Verification items for the finished model (mm, model axes). Face numbers are marked on the shaded views. A direction names the side the tool comes from. Round coordinates to 2 decimals unless told otherwise and drop trailing zeros. Write each loop counter-clockwise with the first axis right and the second up, starting at its lowest first coordinate (ties: lowest second). Pieces come first, ordered by that corner, then holes. Notation, with made-up numbers: (48.5, 85.25) - (106.5, 85.25) arc R27 ccw to (106.5, 118.25) - close; hole circle Ø4 at (24, 41). An arc over 180 degrees is marked (long way). Answer as a JSON object with one key per item and string values. Group by question number.
1) Section check A-A (y = 35). Enter the section's corners in (x, z).
2) Thickness scan on line 1 (X direction, y = 65, z = 3.25); line 2 (Y direction, x = 58, z = 3); line 3 (Y direction, x = -76, z = 10). Record the ranges inside material, lowest first.
3) Mould release check, pull along X, two halves, no side actions. Record for the marked faces 4, 5 and 6: +X half, -X half, draft (parallel to the pull), parting line (faces both ways), or undercut.
4) Section check B-B (x = 58). State how many separate pieces and enclosed holes the cut face has, then the cut area to 3 significant figures.
5) Go/stop test with flat-tipped pins: pin 1 Ø11.5 at (x, y) = (16, 79) entering from +Z; pin 2 Ø6.5 at (x, y) = (16, -43) entering from -Z; pin 3 Ø9 at (y, z) = (-80, 10) entering from +X. Record where each tip stops, or that it passes through.
6) Set-up check for the marked faces 1, 2 and 3: record each of +Z, -Z, +X, -X, +Y, -Y from which the full face is reachable in a straight line by a thin tool's end or side.
```python
from build123d import *

# Parameters (mm, degrees)
SKETCH_1_W                   = 186
SKETCH_1_H                   = 200
EXTRUDE_1_DEPTH              = 20
HOLE_WIZARD_M12_1_AT_2_COUNT = 2
HOLE_WIZARD_M12_1_AT_2_PITCH = 80
HOLE_WIZARD_M12_1_AT_3_COUNT = 2
HOLE_WIZARD_M12_1_AT_3_PITCH = 160
SKETCH_4_W                   = 44
SKETCH_4_H                   = 200
CUT_EXTRUDE_1_DEPTH          = 2
HOLE_WIZARD_2_D              = 5.5
HOLE_WIZARD_2_CBORE_D        = 10
HOLE_WIZARD_2_CBORE_DEPTH    = 6.5
HOLE_WIZARD_2_2_D            = 6.6
HOLE_WIZARD_2_2_CBORE_D      = 11
HOLE_WIZARD_2_2_CBORE_DEPTH  = 6.8
HOLE_WIZARD_M4_1_D           = 3.3
HOLE_WIZARD_M4_1_DEPTH       = 10.1
HOLE_WIZARD_M4_1_TIP         = 0.991420021
CUT_EXTRUDE_2_DEPTH          = 139.018114753
HOLE_WIZARD_M4_2_D           = 3.3
HOLE_WIZARD_M4_2_DEPTH       = 10.1
HOLE_WIZARD_M4_2_TIP         = 0.991420021
HOLE_WIZARD_M3_1_D           = 2.5
HOLE_WIZARD_M3_1_DEPTH       = 7.5
HOLE_WIZARD_M3_1_TIP         = 0.751075774
HOLE_WIZARD_1_D              = 25
HOLE_WIZARD_M6_1_D           = 5


with BuildPart() as part:
    # 草图1 → 凸台-拉伸1 (new body)
    with BuildSketch(Plane.XY):
        Rectangle(SKETCH_1_W, SKETCH_1_H)
    extrude(amount=EXTRUDE_1_DEPTH)

    # 草图2 → M12 螺纹孔1 (revolve, cut)
    with BuildSketch(Plane(origin=(-93, 80, 10), x_dir=(0, 0, 1), z_dir=(0, 1, 0))):
        Polygon((0, 0), (0, 30.064389157), (5.1, 27), (5.1, 0), align=None)
    hole_wizard_m12_1 = revolve(axis=Axis((-99.35, 80, 10), (1, 0, 0)), mode=Mode.SUBTRACT)

    # M12 螺纹孔1 at 2: M12 螺纹孔1 ×2
    with Locations(*[(0, -i * HOLE_WIZARD_M12_1_AT_2_PITCH, 0) for i in range(1, HOLE_WIZARD_M12_1_AT_2_COUNT)]):
        add(hole_wizard_m12_1, mode=Mode.SUBTRACT)

    # M12 螺纹孔1 at 3: M12 螺纹孔1 ×2
    with Locations(*[(0, -i * HOLE_WIZARD_M12_1_AT_3_PITCH, 0) for i in range(1, HOLE_WIZARD_M12_1_AT_3_COUNT)]):
        add(hole_wizard_m12_1, mode=Mode.SUBTRACT)

    # 镜向1: M12 螺纹孔1 across plane
    add(hole_wizard_m12_1.mirror(Plane(origin=(0, 0, 0), x_dir=(0, 0, 1), z_dir=(1, 0, 0))), mode=Mode.SUBTRACT)

    # 镜向1 copy 1 sketch → 镜向1 copy 1 (revolve, cut)
    with BuildSketch(Plane(origin=(93, 0, 10), x_dir=(0, 0, 1), z_dir=(0, 1, 0))):
        Polygon((0, 0), (0, -30.064389157), (5.1, -27), (5.1, 0), align=None)
    revolve(axis=Axis((99.35, 0, 10), (1, 0, 0)), mode=Mode.SUBTRACT)

    # 镜向1 copy 2 sketch → 镜向1 copy 2 (revolve, cut)
    with BuildSketch(Plane(origin=(93, -80, 10), x_dir=(0, 0, 1), z_dir=(0, 1, 0))):
        Polygon((0, 0), (0, -30.064389157), (5.1, -27), (5.1, 0), align=None)
    revolve(axis=Axis((99.35, -80, 10), (1, 0, 0)), mode=Mode.SUBTRACT)

    # 草图4 → 切除-拉伸1 (cut)
    with BuildSketch(Plane.XY.offset(20)):
        Rectangle(SKETCH_4_W, SKETCH_4_H)
    extrude(amount=-CUT_EXTRUDE_1_DEPTH, mode=Mode.SUBTRACT)

    # Hole Wizard 2 (through all)
    with Locations(Plane(origin=(0, 0, 0), x_dir=(-1, 0, 0), z_dir=(0, 0, -1))):
        with Locations((16, 79), (16, 43), (-16, 43), (-16, 79), (-16, -79), (-16, -43), (16, -43), (16, -79)):
            CounterBoreHole(HOLE_WIZARD_2_D / 2, HOLE_WIZARD_2_CBORE_D / 2, HOLE_WIZARD_2_CBORE_DEPTH)

    # Hole Wizard 2 2 (through all)
    with Locations(Plane(origin=(0, 0, 0), x_dir=(-1, 0, 0), z_dir=(0, 0, -1))):
        with Locations((-58, 94), (-58, 55), (-58, 16), (-83, 55)):
            CounterBoreHole(HOLE_WIZARD_2_2_D / 2, HOLE_WIZARD_2_2_CBORE_D / 2, HOLE_WIZARD_2_2_CBORE_DEPTH)

    # M4 螺纹孔1
    with Locations(Plane(origin=(0, 100, 0), x_dir=(1, 0, 0), z_dir=(0, 1, 0))):
        with Locations((-80, -10), (80, -10)):
            Hole(HOLE_WIZARD_M4_1_D / 2, depth=HOLE_WIZARD_M4_1_DEPTH)
            with Locations((0, 0, -(HOLE_WIZARD_M4_1_DEPTH + HOLE_WIZARD_M4_1_TIP / 2))):  # 118° drill point
                Cone(0, HOLE_WIZARD_M4_1_D / 2, HOLE_WIZARD_M4_1_TIP, mode=Mode.SUBTRACT)

    # 草图11 → 切除-拉伸2 (cut, through all)
    with BuildSketch(Plane(origin=(0, 0, 0), x_dir=(-1, 0, 0), z_dir=(0, 0, -1))):
        with BuildLine():
            Line((-17, -24), (17, -24))
            ThreePointArc((17, -24), (20.535533906, -22.535533906), (22, -19))
            Line((22, -19), (22, 19))
            ThreePointArc((22, 19), (20.535533906, 22.535533906), (17, 24))
            Line((17, 24), (-17, 24))
            ThreePointArc((-17, 24), (-20.535533906, 22.535533906), (-22, 19))
            Line((-22, 19), (-22, -19))
            ThreePointArc((-22, -19), (-20.535533906, -22.535533906), (-17, -24))
        make_face()
    extrude(amount=-CUT_EXTRUDE_2_DEPTH, mode=Mode.SUBTRACT)

    # M4 螺纹孔2
    with Locations(Plane(origin=(0, 0, 0), x_dir=(-1, 0, 0), z_dir=(0, 0, -1))):
        with Locations((-12.5, 65), (12.5, 65)):
            Hole(HOLE_WIZARD_M4_2_D / 2, depth=HOLE_WIZARD_M4_2_DEPTH)
            with Locations((0, 0, -(HOLE_WIZARD_M4_2_DEPTH + HOLE_WIZARD_M4_2_TIP / 2))):  # 118° drill point
                Cone(0, HOLE_WIZARD_M4_2_D / 2, HOLE_WIZARD_M4_2_TIP, mode=Mode.SUBTRACT)

    # M3 螺纹孔1
    with Locations(Plane.XY.offset(20)):
        with Locations((-32, 70), (-32, -70), (-40, -70), (-40, 70)):
            Hole(HOLE_WIZARD_M3_1_D / 2, depth=HOLE_WIZARD_M3_1_DEPTH)
            with Locations((0, 0, -(HOLE_WIZARD_M3_1_DEPTH + HOLE_WIZARD_M3_1_TIP / 2))):  # 118° drill point
                Cone(0, HOLE_WIZARD_M3_1_D / 2, HOLE_WIZARD_M3_1_TIP, mode=Mode.SUBTRACT)

    # 孔1 (through all)
    with Locations(Plane.XY.offset(20)):
        with Locations((77, 35)):
            Hole(HOLE_WIZARD_1_D / 2)

    # M6 螺纹孔1 (through all)
    with Locations(Plane(origin=(0, 0, 0), x_dir=(-1, 0, 0), z_dir=(0, 0, -1))):
        with Locations((-58, 85)):
            Hole(HOLE_WIZARD_M6_1_D / 2)


solid = part.part
```
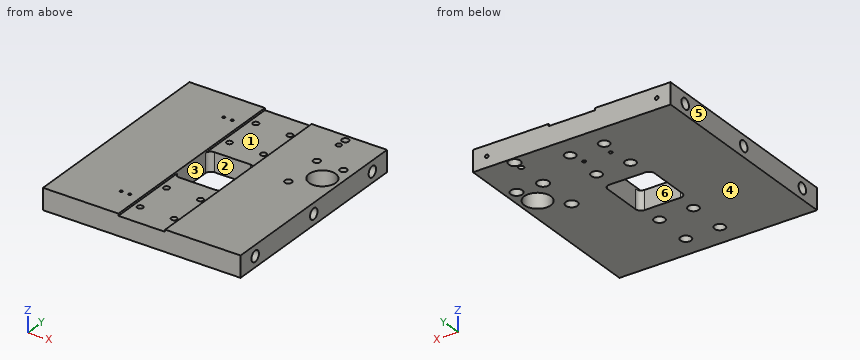
Returned:
{
 "1": {"outline": "(-93, 0) - (64.5, 0) - (64.5, 20) - (22, 20) - (22, 18) - (-22, 18) - (-22, 20) - (-93, 20) - close; (89.5, 0) - (93, 0) - (93, 20) - (89.5, 20) - close"},
 "2": {"line 1": "-93 to -14.15, -10.85 to 10.85, 14.15 to 93", "line 2": "-100 to 10.5, 21.5 to 49.5, 60.5 to 82.5, 87.5 to 88.5, 99.5 to 100", "line 3": "-100 to -85.1, -74.9 to -5.1, 5.1 to 74.9, 85.1 to 100"},
 "3": {"face 4": "draft", "face 5": "-X half", "face 6": "undercut"},
 "4": {"separate pieces": "5", "enclosed holes": "0", "area": "3,410 mm2"},
 "5": {"pin 1": "z = 18", "pin 2": "z = 6.5", "pin 3": "x = 65.64"},
 "6": {"face 1": "+Z, +Y, -Y", "face 2": "+Z, -Z", "face 3": "+Z"}
}
